Design review of the part shown in the three views and the two pictorial views. Dimensions are in mm from the part's minimum x, y and z. A direction names the side the tool comes from. Give positions to 0.01 mm unless a question says otherwise; leave off trailing zeros. Write each loop counter-clockwise with the first axis right and the second up, starting at its lowest first coordinate (ties: lowest second). Pieces come first, ordered by that corner, then holes. Notation, with made-up numbers: (1, 24) -> (45, 24) arc R19 cw to (45, 42) -> close; hole circle Ø1 at (39.5, 57). An arc over 180 degrees is marked (long way). Use CSV: the item, a comma, the result in double quotes.
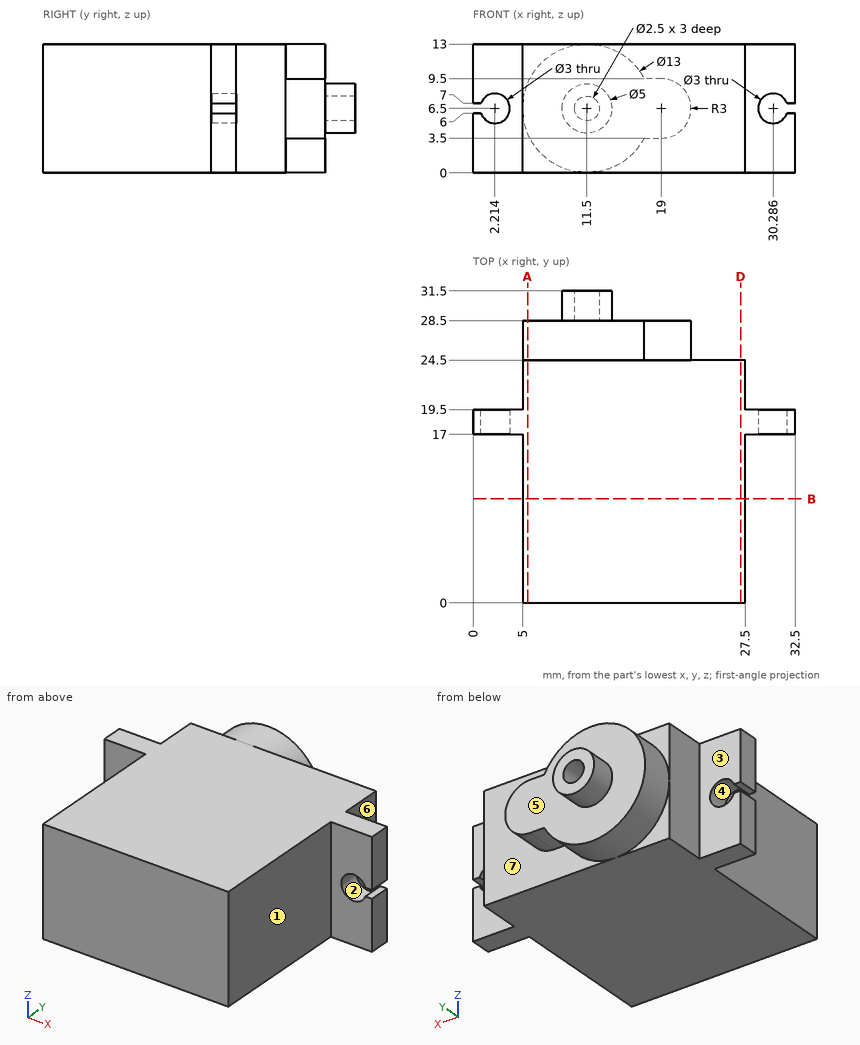
Q1. Consider section B-B (y = 10.5). Write out the cut boundary in (x, z).
Derived:
outline,"(5, 0) -> (27.5, 0) -> (27.5, 13) -> (5, 13) -> close"
Q2. The part is to be moulded in two halves that separate along X. For the marked faces 1, 2, 3 and 4, say which applies: pulls with the +X half, pulls with the -X half, needs draft (parallel to the pull), parting line crosses it, or undercut.
Derived:
face 1,"pulls with the +X half"
face 2,"undercut"
face 3,"needs draft"
face 4,"undercut"
Q3. Machinability: for the marked faces 5, 6 and 7, which of the approach directions +Z, -Z, +X, -X, +Y, -Y give a long, thin tool a straight path to every point of the face, cutting with its end or side? Answer none if there is none.
Derived:
face 5,"+Y"
face 6,"+Z, -Z, +X, +Y"
face 7,"+X, +Y"
Q4. To check wall thickness, follow probe 1 along Z at (x, y) = (11.5, 29.55); probe 2 along Y at (x, z) = (23.5, 11.25); probe 3 along Y at (x, z) = (20.5, 6). State the ranges of each line that lie inside material, in increasing order.
Derived:
probe 1,"z = 4 to 5.25, 7.75 to 9"
probe 2,"y = 0 to 24.5"
probe 3,"y = 0 to 28.5"
Q5. Consider section D-D (x = 27). Write out the cut boundary in (y, z), then the cut area to 4 significant figures.
Derived:
outline,"(0, 0) -> (24.5, 0) -> (24.5, 13) -> (0, 13) -> close"
area,"318.5 mm2"
Q6. Consider section A-A (x = 5.5). Write out the cut boundary in (y, z), then the cut area to 4 significant figures.
Derived:
outline,"(0, 0) -> (24.5, 0) -> (24.5, 4) -> (28.5, 4) -> (28.5, 9) -> (24.5, 9) -> (24.5, 13) -> (0, 13) -> close"
area,"338.5 mm2"
Q7. Insertion check: pin 1 (4 mm diameter, centred on y = 11, z = 7.5, fed in from +X); pin 2 (5.5 mm diameter, centred on y = 23, z = 7, fed in from -X); pin 3 (2 mm diameter, centred on x = 7.5, z = 11.5, fed in from +Y); pin 4 (2.5 mm diameter, centred on x = 2.21, z = 6.5, fed in from +Y). Each pin has a flat end and moves straight along its axis. Give the tip position at first contact, or say it passes through.
Derived:
pin 1,"stops at x = 27.5"
pin 2,"stops at x = 5"
pin 3,"stops at y = 28.5"
pin 4,"passes through"
